```python
from build123d import *

# Parameters (mm, degrees)
EXTRUDECUTONE_DEPTH     = 10.800356134
PATTERNONE_COUNT        = 11
SKETCHHOLE_R            = 23.5
CUT_EXTRUDEA_DEPTH      = 12.050356134
CUT_EXTRUDEA_DEPTH_BACK = 12.050356134
SKETCH_3_OUTSIDE_W      = 129.786
SKETCH_3_OUTSIDE_H      = 128.809
SKETCH_3_OUTSIDE_R      = 37.048512268
CUT_EXTRUDE_4_DEPTH     = 23.100712268
SKETCH_4_R              = 23.5
SKETCH_4_R_2            = 20.5
EXTRUDE_1_DEPTH         = 1.5


with BuildPart() as part:
    # Sketch1 → Revolve 2 (revolve)
    with BuildSketch(Plane.XY):
        with BuildLine():
            Line((-11.050356134, 0), (-11.050356134, 30))
            Line((-11.050356134, 30), (-10.336534907, 30))
            ThreePointArc((-10.336534907, 30), (-8.317543587, 30.836293587), (-7.48125, 32.855284907))
            Line((-7.48125, 32.855284907), (-7.48125, 37.138212268))
            ThreePointArc((-7.48125, 37.138212268), (-6.685622836, 43.788705552), (-4.17925, 50))
            Line((-4.17925, 50), (4.17925, 50))
            ThreePointArc((4.17925, 50), (6.685622836, 43.788705552), (7.48125, 37.138212268))
            Line((7.48125, 37.138212268), (7.48125, 32.855284907))
            ThreePointArc((7.48125, 32.855284907), (8.317543587, 30.836293587), (10.336534907, 30))
            Line((10.336534907, 30), (11.050356134, 30))
            Line((11.050356134, 30), (11.050356134, 0))
            Line((11.050356134, 0), (-11.050356134, 0))
        make_face()
    revolve(axis=Axis((-4, 0, 0), (1, 0, 0)))

    # Sketch2 → ExtrudeCutOne (cut, symmetric)
    with BuildSketch(Plane(origin=(0, 0, 0), x_dir=(0, 0, -1), z_dir=(1, 0, 0))):
        with BuildLine():
            Line((8.716675765, 43.732789559), (9.255531143, 44.765919154))
            ThreePointArc((9.255531143, 44.765919154), (10.574511832, 46.771349182), (12.269067769, 48.471331487))
            ThreePointArc((12.269067769, 48.471331487), (0, 50), (-12.269067769, 48.471331487))
            ThreePointArc((-12.269067769, 48.471331487), (-10.574511832, 46.771349182), (-9.255531143, 44.765919154))
            Line((-9.255531143, 44.765919154), (-8.716675765, 43.732789559))
            ThreePointArc((-8.716675765, 43.732789559), (-7.522276521, 41.726996037), (-6.109966983, 39.868184863))
            ThreePointArc((-6.109966983, 39.868184863), (0, 37.048512268), (6.109966983, 39.868184863))
            ThreePointArc((6.109966983, 39.868184863), (7.522276521, 41.726996037), (8.716675765, 43.732789559))
        make_face()
    extrudecutone = extrude(amount=EXTRUDECUTONE_DEPTH, both=True, mode=Mode.SUBTRACT)

    # PatternOne: ExtrudeCutOne ×11 about axis
    patternone_axis = Axis((0, 0, 0), (1, 0, 0))
    for i in range(1, PATTERNONE_COUNT):
        add(extrudecutone.rotate(patternone_axis, i * 360 / PATTERNONE_COUNT), mode=Mode.SUBTRACT)

    # SketchHole → Cut-ExtrudeA (cut, two sides)
    with BuildSketch(Plane(origin=(0, 0, 0), x_dir=(0, 0, -1), z_dir=(1, 0, 0))) as cut_extrudea_sk:
        Circle(SKETCHHOLE_R)
    extrude(amount=CUT_EXTRUDEA_DEPTH, mode=Mode.SUBTRACT)
    extrude(cut_extrudea_sk.sketch, amount=-CUT_EXTRUDEA_DEPTH_BACK, mode=Mode.SUBTRACT)

    # Sketch 3 outside → Cut-Extrude 4 (cut, through all)
    with BuildSketch(Plane(origin=(11.050356134, 0, 0), x_dir=(0, 0, -1), z_dir=(1, 0, 0))):
        with Locations((0, -0.7645)):
            Rectangle(SKETCH_3_OUTSIDE_W, SKETCH_3_OUTSIDE_H)
        Circle(SKETCH_3_OUTSIDE_R, mode=Mode.SUBTRACT)
    extrude(amount=-CUT_EXTRUDE_4_DEPTH, mode=Mode.SUBTRACT)

    # Sketch 4 → Extrude 1 (add, symmetric)
    with BuildSketch(Plane(origin=(0, 0, 0), x_dir=(0, 0, -1), z_dir=(1, 0, 0))):
        Circle(SKETCH_4_R)
        Circle(SKETCH_4_R_2, mode=Mode.SUBTRACT)
    extrude(amount=EXTRUDE_1_DEPTH, both=True)


solid = part.part
```
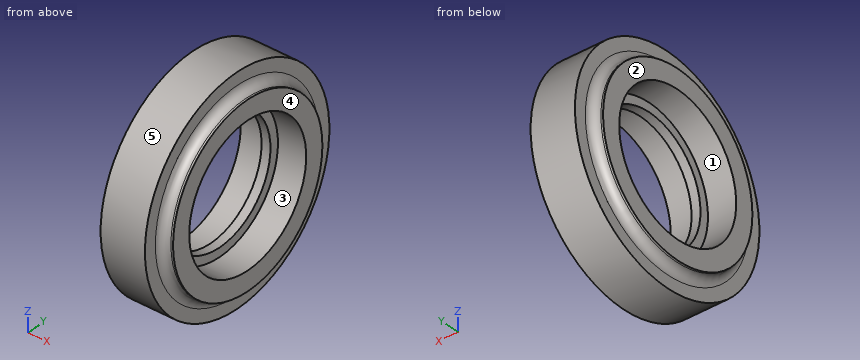
Here's how the part is built. I have some questions about the finished solid (model axes, mm). Face numbers are marked on the shaded views. A direction names the side the tool comes from. Round coordinates to 2 decimals unless told otherwise and drop trailing zeros. Order: outer loops, then holes, each group sorted by start corner. A loop starts at its lowest first (then second) coordinate and runs counter-clockwise, first axis right, second up. Notation, with made-up numbers: (26, 52.25) -> (45, 52.25) arc R17 ccw to (45, 70.25) -> close; hole circle Ø1 at (50, 8). An arc over 180 degrees is marked (long way). Use a Markdown table: item, result. Add a question column.
(1) I need wall thicknesses on line 1 along Y through (x, z) = (4.25, 1); line 2 along Y through (x, z) = (0.1, 0); line 3 along Z through (x, y) = (-5, -4). Which ranges of each line are inside material? Lowest first, please.
(2) Suppose I cut it at D-D, the plane x = 8.5. Please give me the cut outline in (y, z).
(3) Suppose I cut it at A-A, the plane y = 0. Please give me the cut outline in (x, z).
(4) Suppose I cut it at C-C, the plane x = -0.5. Please give me the cut outline in (y, z), and give its area (3 significant figures).
(5) For pin 1 Ø1.5 at (x, y) = (4, -25.5) entering from -Z; pin 2 Ø2 at (x, z) = (-7.5, 16) entering from +Y; pin 3 Ø1 at (x, z) = (-2, -15) entering from +Y; pin 4 Ø24.5 at (y, z) = (0, 0) entering from +X, each with a flat end and sliding along its axis, tell me the tip position at first contact or that it passes through.
(6) For the marked faces 1 and 2, which set-ups out of +Z, -Z, +X, -X, +Y, -Y let a thin tool reach every point of the face, with its end or its side?
(7) If we mould it in two halves opening along Z, with no side actions, what happens to the marked faces 3, 4 and 5? For each: released by +Z, released by -Z, zero draft, split by the parting line, or undercut.
Verdict:
| question | item | result |
|---|---|---|
| 1 | line 1 | -37.04 to -23.48, 23.48 to 37.04 |
| 1 | line 2 | -37.05 to -20.5, 20.5 to 37.05 |
| 1 | line 3 | -36.83 to -23.16, 23.16 to 36.83 |
| 2 | outline | circle Ø61.34 at (0, 0); hole circle Ø47 at (0, 0) |
| 3 | outline | (-11.05, -30) -> (-10.34, -30) arc R2.86 cw to (-7.48, -32.86) -> (-7.48, -37.05) -> (7.48, -37.05) -> (7.48, -32.86) arc R2.86 cw to (10.34, -30) -> (11.05, -30) -> (11.05, -23.5) -> (1.5, -23.5) -> (1.5, -20.5) -> (-1.5, -20.5) -> (-1.5, -23.5) -> (-11.05, -23.5) -> close; (-11.05, 23.5) -> (-1.5, 23.5) -> (-1.5, 20.5) -> (1.5, 20.5) -> (1.5, 23.5) -> (11.05, 23.5) -> (11.05, 30) -> (10.34, 30) arc R2.86 cw to (7.48, 32.86) -> (7.48, 37.05) -> (-7.48, 37.05) -> (-7.48, 32.86) arc R2.86 cw to (-10.34, 30) -> (-11.05, 30) -> close |
| 4 | outline | circle Ø74.1 at (0, 0); hole circle Ø41 at (0, 0) |
| 4 | area | 2,990 mm2 |
| 5 | pin 1 | z = -27.57 |
| 5 | pin 2 | y = 33.88 |
| 5 | pin 3 | y = 34.09 |
| 5 | pin 4 | through |
| 6 | face 1 | -X |
| 6 | face 2 | +Z, -Z, -X, +Y, -Y |
| 7 | face 3 | undercut |
| 7 | face 4 | zero draft |
| 7 | face 5 | split by the parting line |
